```python
from build123d import *

# Parameters (mm, degrees)
SKETCH1_R           = 6
SKETCH1_R_2         = 5
BOSS_EXTRUDE1_DEPTH = 20
SKETCH2_W           = 17.887562732
SKETCH2_H           = 2.1
CUT_EXTRUDE1_DEPTH  = 5
FILLET2_SIZE        = 1
FILLET2_SIZE_2      = 3


with BuildPart() as part:
    # Sketch1 → Boss-Extrude1 (new body)
    with BuildSketch(Plane.XY):
        Circle(SKETCH1_R)
        Circle(SKETCH1_R_2, mode=Mode.SUBTRACT)
    extrude(amount=BOSS_EXTRUDE1_DEPTH)

    # Sketch2 → Cut-Extrude1 (cut)
    with BuildSketch(Plane(origin=(0, 0, 0), x_dir=(-1, 0, 0), z_dir=(0, 0, -1))):
        Rectangle(SKETCH2_W, SKETCH2_H)
    extrude(amount=-CUT_EXTRUDE1_DEPTH, mode=Mode.SUBTRACT)

    # Fillet2
    # a fillet whose section is not a circle: 3, 1 mm, written as the material it takes off along each edge
    with BuildSketch(Plane(origin=(0, 0, 0), x_dir=(-0.2768991619260433, 0.9608989822685082, 0), z_dir=(0.9608989822685082, 0.2768991619260433, 0))) as fillet2_piece_1:
        with BuildLine():
            Bezier((5 + FILLET2_SIZE, 0), (5, 0), (5, FILLET2_SIZE_2), weights=[1, 0.707106781, 1])
            Line((5, FILLET2_SIZE_2), (5, 0))
            Line((5, 0), (5 + FILLET2_SIZE, 0))
        make_face()
    revolve(axis=Axis((0, 0, 0), (0, 0, 1)), revolution_arc=327.849552319, mode=Mode.SUBTRACT)
    with BuildSketch(Plane(origin=(0, 0, 0), x_dir=(0.2768991619260793, -0.9608989822684979, 0), z_dir=(-0.9608989822684979, -0.2768991619260793, 0))) as fillet2_piece_2:
        with BuildLine():
            Bezier((5 + FILLET2_SIZE, 0), (5, 0), (5, FILLET2_SIZE_2), weights=[1, 0.707106781, 1])
            Line((5, FILLET2_SIZE_2), (5, 0))
            Line((5, 0), (5 + FILLET2_SIZE, 0))
        make_face()
    revolve(axis=Axis((0, 0, 0), (0, 0, 1)), revolution_arc=327.849552319, mode=Mode.SUBTRACT)


solid = part.part
```
Verification items for the finished model (mm, model axes). A direction names the side the tool comes from. Round coordinates to 2 decimals unless told otherwise and drop trailing zeros. Write each loop counter-clockwise with the first axis right and the second up, starting at its lowest first coordinate (ties: lowest second). Pieces come first, ordered by that corner, then holes.
1. Section check A-A on y = 0. Enter the section's corners in (x, z).
2. Access from +Z, -Z, +X, -X, +Y, -Y to the whole of each face (thin tool, end or side, straight path). Record for faces 1 (the flat face through (5.4, 1.05, 2.5)), 2 (the cylindrical face through (4.619, -1.915, 11.381)).
3. Scan lines: L1, parallel to Y at x = 0, z = 10; L2, parallel to Y at x = -1.5, z = 9.5. Record each from-to range of solid material in increasing order.
4. Draft check along Y on faces 3 (the flat face through (5.4, -1.05, 2.5)), 4 (the cylindrical face through (5.723, 1.802, 9.86)), 5 (the flat face through (-5.4, 1.05, 3)), 6 (the flat face through (-4, 4, 20)). Enter one of: +Y half, -Y half, draft (parallel to the pull), parting line (faces both ways), or undercut.
5. Section check B-B on z = 3.25. Enter the section's corners in (x, y), plus the area to 3 significant figures.
6. Gauge pin test, flat ends, axial feed: P1, Ø5, axis at x = 1, y = 1.5, coming from the +Z side; P2, Ø1.1, axis at x = 5, z = 3.5, coming from the +Y side; P3, Ø6, axis at x = -3.5, z = 3.5, coming from the +Y side; P4, Ø4, axis at y = 4, z = 15.5, coming from the +X side. Record the tip position at first contact, or that the pin passes through.
7. Section check C-C on z = 9. Enter the section's corners in (x, y), plus the area to 3 significant figures.
Answer:
1. outline: (-6, 5) - (-5, 5) - (-5, 20) - (-6, 20) - close; (5, 5) - (6, 5) - (6, 20) - (5, 20) - close
2. face 1: -Z, +X, -X
2. face 2: +Z, -Z
3. L1: y = -6 to -5, 5 to 6
3. L2: y = -5.81 to -4.77, 4.77 to 5.81
4. face 3: undercut
4. face 4: parting line
4. face 5: undercut
4. face 6: draft
5. outline: (-5.91, -1.05) arc R6 ccw to (5.91, -1.05) - (4.89, -1.05) arc R5 cw to (-4.89, -1.05) - close; (-5.91, 1.05) - (-4.89, 1.05) arc R5 cw to (4.89, 1.05) - (5.91, 1.05) arc R6 ccw to start
5. area: 30.3 mm2
6. P1: passes through
6. P2: stops at y = 4.02
6. P3: stops at y = 5.98
6. P4: stops at x = 5.66
7. outline: circle Ø12 at (0, 0); hole circle Ø10 at (0, 0)
7. area: 34.6 mm2
